```python
from build123d import *

# Parameters (mm, degrees)
EXTRUDE_1_DEPTH = 220
EXTRUDE_2_DEPTH = 1.6
FILLET_1_R      = 1.6
FILLET_2_R      = 3


with BuildPart() as part:
    # Sketch 1 → Extrude 1 (new body)
    with BuildSketch(Plane.XY):
        with BuildLine():
            ThreePointArc((8.6, 238.845221849), (7.800043744, 238.872684327), (7, 238.897467546))
            Line((7, 238.897467546), (7, 237.296776211))
            ThreePointArc((7, 237.296776211), (7.800044336, 237.271825779), (8.6, 237.244178011))
            Line((8.6, 237.244178011), (8.6, 238.845221849))
        make_face()
        with BuildLine():
            ThreePointArc((8.6, 237.244178011), (7.800044336, 237.271825779), (7, 237.296776211))
            Line((7, 237.296776211), (7, 34.292856399))
            ThreePointArc((7, 34.292856399), (7.802144981, 34.119298552), (8.6, 33.926980414))
            Line((8.6, 33.926980414), (8.6, 237.244178011))
        make_face()
        with BuildLine():
            ThreePointArc((224.497758474, 81.986318617), (140.480675298, 193.355061656), (8.6, 238.845221849))
            Line((8.6, 238.845221849), (8.6, 237.244178011))
            ThreePointArc((8.6, 237.244178011), (139.540218894, 192.060634465), (222.975075299, 81.491568862))
            Line((222.975075299, 81.491568862), (224.497758474, 81.986318617))
        make_face()
        with BuildLine():
            ThreePointArc((8.6, 33.926980414), (7.802144981, 34.119298552), (7, 34.292856399))
            Line((7, 34.292856399), (7, 32.658230203))
            ThreePointArc((7, 32.658230203), (7.802367665, 32.475884265), (8.6, 32.273828406))
            Line((8.6, 32.273828406), (8.6, 33.926980414))
        make_face()
        with BuildLine():
            ThreePointArc((29.608929649, 18.663099556), (20.57248383, 28.315594803), (8.6, 33.926980414))
            Line((8.6, 33.926980414), (8.6, 32.273828406))
            ThreePointArc((8.6, 32.273828406), (19.632027427, 27.021167612), (28.03668866, 18.152247491))
            Line((28.03668866, 18.152247491), (29.608929649, 18.663099556))
        make_face()
        with BuildLine():
            ThreePointArc((30.45132558, 17.254471027), (30.038385828, 17.963723914), (29.608929649, 18.663099556))
            Line((29.608929649, 18.663099556), (28.03668866, 18.152247491))
            ThreePointArc((28.03668866, 18.152247491), (28.475337148, 17.456092756), (28.896703685, 16.749343753))
            Line((28.896703685, 16.749343753), (30.45132558, 17.254471027))
        make_face()
        with BuildLine():
            ThreePointArc((223.51952635, 79.986132174), (223.248569783, 80.739309445), (222.975075299, 81.491568862))
            Line((222.975075299, 81.491568862), (29.608929649, 18.663099556))
            ThreePointArc((29.608929649, 18.663099556), (30.038385828, 17.963723914), (30.45132558, 17.254471027))
            Line((30.45132558, 17.254471027), (223.51952635, 79.986132174))
        make_face()
        with BuildLine():
            ThreePointArc((225.041874276, 80.480772999), (224.77107692, 81.234001379), (224.497758474, 81.986318617))
            Line((224.497758474, 81.986318617), (222.975075299, 81.491568862))
            ThreePointArc((222.975075299, 81.491568862), (223.248569783, 80.739309445), (223.51952635, 79.986132174))
            Line((223.51952635, 79.986132174), (225.041874276, 80.480772999))
        make_face()
    extrude(amount=EXTRUDE_1_DEPTH)

    # Sketch 1_3 → Extrude 2 (add)
    with BuildSketch(Plane.XY):
        with BuildLine():
            ThreePointArc((222.975075299, 81.491568862), (139.540218894, 192.060634465), (8.6, 237.244178011))
            Line((8.6, 237.244178011), (8.6, 33.926980414))
            ThreePointArc((8.6, 33.926980414), (20.57248383, 28.315594803), (29.608929649, 18.663099556))
            Line((29.608929649, 18.663099556), (222.975075299, 81.491568862))
        make_face()
    extrude(amount=EXTRUDE_2_DEPTH)

    # Fillet 1
    fillet_1_edges = [part.edges().sort_by_distance(p)[0] for p in [
        (222.975075299, 81.491568862, 110.8),
        (8.6, 237.244178011, 110.8),
        (8.6, 33.926980414, 110.8),
        (29.608929649, 18.663099556, 110.8),
    ]]
    fillet(fillet_1_edges, radius=FILLET_1_R)

    # Fillet 2
    fillet_2_edges = [part.edges().sort_by_distance(p)[0] for p in [
        (7, 32.658230203, 110),
        (7, 238.897467546, 110),
        (225.041874276, 80.480772999, 110),
        (28.896703685, 16.749343753, 110),
    ]]
    fillet(fillet_2_edges, radius=FILLET_2_R)


solid = part.part
```
Geometry: final body of the model. Coordinates: model frame, mm. A direction names the side the tool comes from. Round coordinates to 2 decimals unless told otherwise and drop trailing zeros. Order: outer loops, then holes, each group sorted by start corner. A loop starts at its lowest first (then second) coordinate and runs counter-clockwise, first axis right, second up. Notation, with made-up numbers: (61, 70.25) -> (110, 70.25) arc R26 cw to (110, 97.25) -> close; hole circle Ø1 at (48.25, 72.25). An arc over 180 degrees is marked (long way). Use one line per item in the form item = value.
(1) Ray query, probe 1 along Z at (x, y) = (56.5, 87); probe 2 along Y at (x, z) = (169, 136.5); probe 3 along Y at (x, z) = (196.5, 44). Return the intervals inside material, ascending. Write a range as [from, to].
Results list:
probe_1 = [0, 1.6]
probe_2 = [62.27, 63.95], [166.73, 169]
probe_3 = [71.21, 72.89], [133.22, 136.05]
(2) Section A-A on x = 130. Return loops of the section in (y, z).
Results list:
outline = (49.6, 0) -> (200.55, 0) -> (200.55, 220) -> (198.64, 220) -> (198.64, 1.6) -> (51.28, 1.6) -> (51.28, 220) -> (49.6, 220) -> close
(3) First-contact query: pin 1 Ø4 at (x, z) = (89, 190.5) entering from +Y; pin 2 Ø4 at (x, z) = (110.5, 120.5) entering from -Y; pin 3 Ø2 at (y, z) = (137.5, 126.5) entering from +X. Flat tips, straight axial feed; report the tip coordinate or a pass-through.
Results list:
pin_1 = 222.6
pin_2 = 42.61
pin_3 = 196.19
(4) Section B-B on y = 157. Return loops of the section in (x, z).
Results list:
outline = (7, 0) -> (180.2, 0) -> (180.2, 220) -> (178.07, 220) -> (178.07, 1.6) -> (8.6, 1.6) -> (8.6, 220) -> (7, 220) -> close
(5) Access query for faces 1 (the face through (142.06, 192.2, 108.46)), 2 (the face through (127.416, 50.443, 109.271)). Directions: +Z, -Z, +X, -X, +Y, -Y. A direction counts if a zero-diameter tool reaches every point of the face in a straight line with its end or side. Return the directions, or none.
Results list:
face_1 = +Z, -Z, +X, +Y
face_2 = +Z
(6) Draft query along Y for faces 3 (the face through (19.499, 27.117, 108.46)), 4 (the face through (90, 130, 0)), 5 (the face through (21, 28, 109)), 6 (the face through (8.6, 134, 109)). Return one class per face: pulls with the +Y half, pulls with the -Y half, needs draft (parallel to the pull), parting line crosses it, or undercut.
Results list:
face_3 = pulls with the -Y half
face_4 = needs draft
face_5 = undercut
face_6 = undercut
